Build history of the part. All positions in model axes, mm. Face numbers are marked on the shaded views. A direction names the side the tool comes from. Coordinates: 2 decimals unless noted, no trailing zeros. Write each loop counter-clockwise with the first axis right and the second up, starting at its lowest first coordinate (ties: lowest second). Pieces come first, ordered by that corner, then holes. Notation, with made-up numbers: M 11,71 L 54,71 A21 ccw 54,98 Z; hole C -29.75,14.25 d6. An arc over 180 degrees is marked long. Use CSV: the item, a comma, the result in double quotes. Start each with the question number.
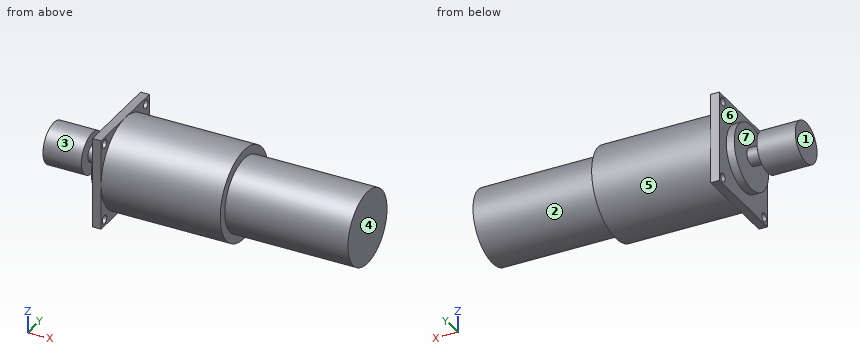
```python
from build123d import *

# Parameters (mm, degrees)
ESBO_O2_W                = 42
ESBO_O2_H                = 42
RESSALTO_EXTRUS_O1_DEPTH = 4
ESBO_O3_R                = 2
CORTE_EXTRUS_O1_DEPTH    = 4


with BuildPart() as part:
    # Esboço1 → Revolução1 (revolve)
    with BuildSketch(Plane.XY):
        Polygon((-29, 0), (-29, 9.5), (-11.2, 9.5), (-11.2, 4), (-3.7, 4), (-3.7, 15), (0, 15), (0, 21), (59.1, 21), (59.1, 17), (116.1, 17), (116.1, 0), align=None)
    revolve(axis=Axis((0, 0, 0), (1, 0, 0)))

    # Esboço2 → Ressalto-extrusão1 (add)
    with BuildSketch(Plane.ZY):
        Rectangle(ESBO_O2_W, ESBO_O2_H)
    extrude(amount=-RESSALTO_EXTRUS_O1_DEPTH)

    # Esboço3 → Corte-extrusão1 (cut)
    with BuildSketch(Plane(origin=(4, 0, 0), x_dir=(0, 0, -1), z_dir=(1, 0, 0))):
        with Locations((-18, 18)):
            Circle(ESBO_O3_R)
        with Locations((-18, -18)):
            Circle(ESBO_O3_R)
        with Locations((18, -18)):
            Circle(ESBO_O3_R)
        with Locations((18, 18)):
            Circle(ESBO_O3_R)
    extrude(amount=-CORTE_EXTRUS_O1_DEPTH, mode=Mode.SUBTRACT)


solid = part.part
```
1. Slice it at B-B (z = 18.5). List the corners of the cut face in (x, y).
2. Slice it at C-C (z = -7.5). List the corners of the cut face in (x, y), and give its area (3 significant figures).
3. Drill centre lines: line 1 along Y through (x, z) = (2.8, 18); line 2 along X through (y, z) = (7.5, -4.5); line 3 along X through (y, z) = (7, -10.5). Where is each one in solid material? Low to high. Write a range as from..to.
4. Slice it at D-D (x = 50). List the corners of the cut face in (y, z), and give its area (3 significant figures).
5. Flat gauge pins, fed straight in: pin 1 (2 mm diameter, centred on y = -13.5, z = -15, fed in from +X); pin 2 (6.5 mm diameter, centred on y = -18, z = 18, fed in from +X); pin 3 (3 mm diameter, centred on x = 80, y = -16, fed in from +Z). Where does each tip first touch, or does it go through?
6. Pull direction X, two halves, no side cores. Call the marked faces 4, 5, 6 and 7: pulls with the +X half, pulls with the -X half, needs draft (parallel to the pull), parting line crosses it, or undercut.
7. Slice it at A-A (y = -6). List the corners of the cut face in (x, z), and give its area (3 significant figures).
8. 3-axis set-ups, long thin cutter, end or side, ignore diameter. For the marked faces 1, 2 and 3: which of +Z, -Z, +X, -X, +Y, -Y reach the whole face in a straight line?
Established:
1,outline,"M 0,-21 L 4,-21 L 4,-19.94 L 0,-19.94 Z; M 0,-16.06 L 4,-16.06 L 4,-9.94 L 59.1,-9.94 L 59.1,9.94 L 4,9.94 L 4,16.06 L 0,16.06 Z; M 0,19.94 L 4,19.94 L 4,21 L 0,21 Z"
2,outline,"M -29,-5.83 L -11.2,-5.83 L -11.2,5.83 L -29,5.83 Z; M -3.7,-12.99 L 0,-12.99 L 0,-21 L 4,-21 L 4,-19.62 L 59.1,-19.62 L 59.1,-15.26 L 116.1,-15.26 L 116.1,15.26 L 59.1,15.26 L 59.1,19.62 L 4,19.62 L 4,21 L 0,21 L 0,12.99 L -3.7,12.99 Z"
2,area,"4,370 mm2"
3,line 1,"y = -21..-20, -16..16, 20..21"
3,line 2,"x = -29..-11.2, -3.7..116.1"
3,line 3,"x = -3.7..116.1"
4,outline,"C 0,0 d42"
4,area,"1,390 mm2"
5,pin 1,"stops at x = 59.1"
5,pin 2,"stops at x = 4"
5,pin 3,"stops at z = 8.87"
6,face 4,"pulls with the +X half"
6,face 5,"needs draft"
6,face 6,"pulls with the -X half"
6,face 7,"undercut"
7,outline,"M -29,-7.37 L -11.2,-7.37 L -11.2,7.37 L -29,7.37 Z; M -3.7,-13.75 L 0,-13.75 L 0,-21 L 4,-21 L 4,-20.12 L 59.1,-20.12 L 59.1,-15.91 L 116.1,-15.91 L 116.1,15.91 L 59.1,15.91 L 59.1,20.12 L 4,20.12 L 4,21 L 0,21 L 0,13.75 L -3.7,13.75 Z"
7,area,"4,560 mm2"
8,face 1,"+Z, -Z, -X, +Y, -Y"
8,face 2,"+X"
8,face 3,"-X"
